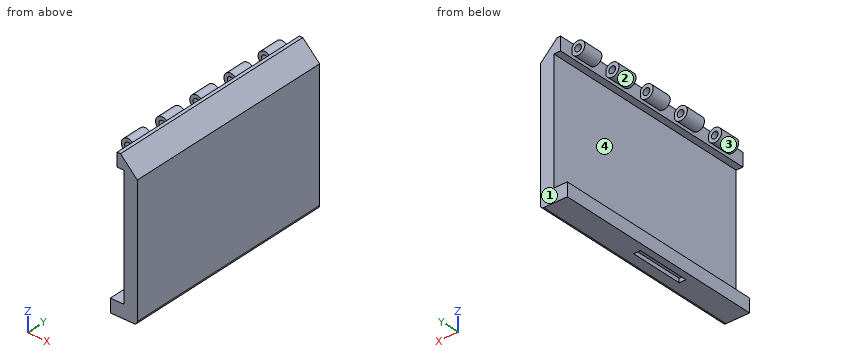
Autodesk Inventor part; units mm, degrees
ref_plane "Work Plane1" through (0, 19.05, 0) normal (0, -1, 0) x (1, 0, 0)
ref_plane "YZ Plane" through (0, 0, 0) normal (1, 0, 0) x (0, 1, 0)
ref_plane "XZ Plane" through (0, 0, 0) normal (0, 1, 0) x (-1, 0, 0)
sketch "Sketch1" plane through (0, 0, 0) normal (1, 0, 0) x (0, 1, 0)
  line L0 (0, 0) -> (203.2, 0)
  line L1 (203.2, 0) -> (203.2, -152.4)
  line L2 (203.2, -152.4) -> (0, -152.4)
  line L3 (0, -152.4) -> (0, 0)
  dimension "d0" = 203.2
  dimension "d1" = 152.4
extrude "Extrusion1" add sketch "Sketch1" along normal blind 12.7
sketch "Sketch2" plane through (0, 0, 0) normal (-1, 0, 0) x (0, 0, 1)
  line L0 (-152.4, 0) -> (-152.4, 203.2)
  line L1 (-152.4, 203.2) -> (0, 203.2)
  line L2 (-152.4, 0) -> (-139.7, 0)
  line L3 (-139.7, 0) -> (-139.7, 203.2)
  line L4 (-139.7, 203.2) -> (-152.4, 203.2)
  line L5 (-152.4, 203.2) -> (-152.4, 0)
  point P0 (0, 0)
  dimension "d4" = 12.7
extrude "Extrusion2" add sketch "Sketch2" along normal blind 12.7
fillet "Fillet1" radius 3.175 1 edges at (12.7, 101.6, -152.4)
sketch "Sketch3" plane through (0, 0, 0) normal (0, -1, 0) x (1, 0, 0)
  line L0 (0, 0) -> (0, -12.7)
  line L1 (0, -12.7) -> (0, -25.4)
  line L2 (0, -12.7) -> (-6.35, -12.7)
  line L3 (-6.35, -12.7) -> (-6.35, -25.4)
  line L4 (-6.35, -25.4) -> (0, -25.4)
  dimension "d8" = 12.7
  dimension "d9" = 12.7
  dimension "d10" = 6.35
  dimension "d11" = 90
extrude "Extrusion3" add sketch "Sketch3" against normal up to surface (203.2 mm away)
ref_plane "Work Plane1" through (0, 19.05, 0) normal (0, -1, 0) x (1, 0, 0)
sketch "Sketch4" plane through (0, 19.05, 0) normal (0, -1, 0) x (1, 0, 0)
  line L0 (0, -19.05) -> (-12.065, -19.05)
  circle A0 centre (-12.065, -19.05) radius 3.175
  circle A1 centre (-12.065, -19.05) radius 6.35
  point P0 (0, 0)
  dimension "d15" = 12.065
  dimension "d16" = 6.35
  dimension "d17" = 12.7
  dimension "d18" = 19.05
  dimension "d19" = 19.05
extrude "Extrusion4" add sketch "Sketch4" against normal blind 19.05
pattern_linear "Rectangular Pattern1" count 5 spacing 38.1 along (0, 1, 0) of "Extrusion4"
sketch "Sketch5" plane through (0, 203.2, 0) normal (0, 1, 0) x (1, 0, 0)
  line L0 (0, 0) -> (12.7, 0)
  line L1 (12.7, 0) -> (12.7, 12.7)
  line L2 (12.7, 12.7) -> (0, 12.7)
  line L3 (0, 12.7) -> (0, 0)
  line L4 (12.7, 149.225) -> (12.7, 0)
extrude "Extrusion5" cut sketch "Sketch5" against normal blind 203.2
chamfer "Chamfer2" distance 15.875 angle 45 1 edges at (12.7, 101.6, -12.7)
sketch "Sketch6" plane through (-12.7, 0, -152.4) normal (0, 0, -1) x (-1, 0, 0)
  line L0 (0, 0) -> (0, 63.5)
  line L1 (0, 63.5) -> (-6.35, 63.5)
  line L2 (-12.7, 0) -> (-12.7, 203.2)
  line L3 (-6.35, 63.5) -> (-12.7, 63.5)
  line L4 (-12.7, 63.5) -> (-12.7, 114.3)
  line L5 (-12.7, 114.3) -> (-6.35, 114.3)
  line L6 (-6.35, 114.3) -> (-6.35, 63.5)
  dimension "d35" = 63.5
  dimension "d37" = 6.35
  dimension "d38" = 50.8
extrude "Extrusion6" cut sketch "Sketch6" against normal blind 3.81
properties part number "PhoneSafeDoor(H)"
CAD build for the part. Positions are in the model's coordinates, mm. Face numbers are marked on the shaded views. Round coordinates to 2 decimals unless told otherwise and drop trailing zeros. Order: outer loops, then holes, each group sorted by start corner. A loop starts at its lowest first (then second) coordinate and runs counter-clockwise, first axis right, second up.
Q1. Drop flat-ended pins along their axis: pin 1 (4 mm diameter, centred on y = 81, z = -150, fed in from +X); pin 2 (4 mm diameter, centred on y = 83, z = -150, fed in from -X); pin 3 (3.5 mm diameter, centred on x = -10.5, z = -18, fed in from -Y); pin 4 (3.5 mm diameter, centred on x = -12, z = -21.5, fed in from +Y). Give the stop position or say it passes through.
Q2. Two-plate mould, pull along X, no slides. Class the marked faces 1, 2, 3 and 4: pulls with the +X half, pulls with the -X half, needs draft (parallel to the pull), parting line crosses it, or undercut.
Q3. Slice it at A-A (y = 61). Write the cut outline in (x, z) (3 decimals).
Q4. Slice it at C-C (z = -41). Write the cut outline in (x, y).
Q5. Slice it at B-B (y = 117). Write the cut outline in (x, z) (3 decimals).
Q6. Wall check: L1, parallel to Z at x = -12, y = 175.5; L2, parallel to Z at x = -4, y = 189; L3, parallel to Z at x = -2, y = 101.5 (3 decimals). Give the ranges that are in metal, low to high.
Q7. Slice it at D-D (z = -19.05). State how many separate pieces and enclosed holes the cut face has, and give its area (3 significant figures).
Results below:
1. pin 1: stops at x = 12.7
1. pin 2: stops at x = -12.7
1. pin 3: stops at y = 19.05
1. pin 4: stops at y = 190.5
2. face 1: needs draft
2. face 2: undercut
2. face 3: undercut
2. face 4: pulls with the -X half
3. outline: (-12.7, -152.4) - (9.525, -152.4) arc R3.175 ccw to (12.7, -149.225) - (12.7, -28.575) - (-3.175, -12.7) - (-6.35, -12.7) - (-6.35, -16.282) arc R6.35 ccw (long way) to (-6.35, -21.818) - (-6.35, -25.4) - (0, -25.4) - (0, -139.7) - (-12.7, -139.7) - close; hole circle Ø6.35 at (-12.065, -19.05)
4. outline: (0, 0) - (12.7, 0) - (12.7, 203.2) - (0, 203.2) - close
5. outline: (-12.7, -152.4) - (9.525, -152.4) arc R3.175 ccw to (12.7, -149.225) - (12.7, -28.575) - (-3.175, -12.7) - (-6.35, -12.7) - (-6.35, -25.4) - (0, -25.4) - (0, -139.7) - (-12.7, -139.7) - close
6. L1: z = -152.4 to -139.7, -25.4 to -22.22, -15.88 to -12.7
6. L2: z = -152.4 to -139.7, -25.4 to -12.7
6. L3: z = -148.59 to -139.7, -25.4 to -13.875
7. separate pieces: 6
7. enclosed holes: 0
7. area: 2,480 mm2
